Geometry: final body of the model. Coordinates: model frame, mm. Round coordinates to 2 decimals unless told otherwise and drop trailing zeros. Write each loop counter-clockwise with the first axis right and the second up, starting at its lowest first coordinate (ties: lowest second). Pieces come first, ordered by that corner, then holes. Notation, with made-up numbers: M 77.25,64 L 92.25,64 A33 cw 92.25,98 Z; hole C 27.5,77 d7. An arc over 180 degrees is marked long. Use one line per item in the form item = value. Start each with the question number.
Item 1: Section query A-A (z = 8.5). Return loops of the section in (x, y).
Item 2: Section query C-C (y = -6.5). Return loops of the section in (x, z), and give its area (3 significant figures).
Item 3: Pin query (flat end, axial travel): pin 1 Ø1 at (y, z) = (-99.5, 6) entering from -X; pin 2 Ø5 at (y, z) = (-77, 16) entering from +X; pin 3 Ø8 at (y, z) = (-72.5, 12) entering from -X. Return the tip coordinate at first contact, or that it passes through.
Item 4: Section query B-B (x = -91.5). Return loops of the section in (y, z).
Item 5: Ray query, probe 1 along Y at (x, z) = (108.5, 17); probe 2 along Y at (x, z) = (-93, 7.5); probe 3 along X at (y, z) = (-69, 2.25). Return the intervals inside material, ascending.
from build123d import *

# Parameters (mm, degrees)
BOSS_EXTRUDE1_DEPTH = 19.05
FILLET1_R           = 50.8


with BuildPart() as part:
    # Sketch1 → Boss-Extrude1 (new body)
    with BuildSketch(Plane.XY):
        with BuildLine():
            Line((-127, 0), (127, 0))
            Line((127, 0), (76.2, -101.6))
            ThreePointArc((76.2, -101.6), (0, -122.017728463), (-76.2, -101.6))
            Line((-76.2, -101.6), (-127, 0))
        make_face()
    extrude(amount=BOSS_EXTRUDE1_DEPTH)

    # Fillet1
    fillet1_edges = [part.edges().sort_by_distance(p)[0] for p in [
        (76.2, -101.6, 9.525),
        (-76.2, -101.6, 9.525),
    ]]
    fillet(fillet1_edges, radius=FILLET1_R)


solid = part.part
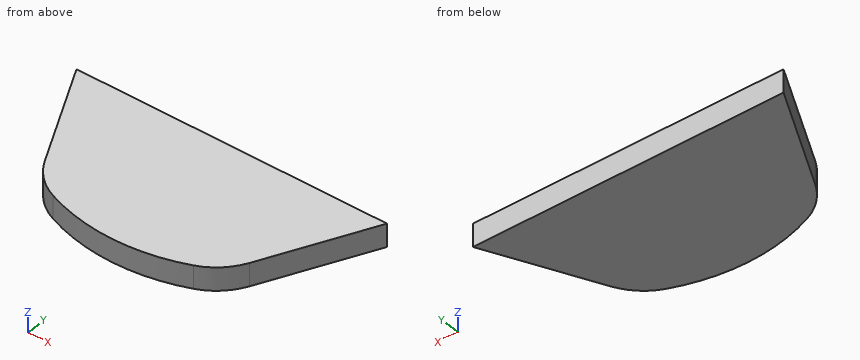
Working result:
q1.outline = M -127,0 L -83.79,-86.42 A50.8 ccw -57.53,-110.74 A152.4 ccw 57.53,-110.74 A50.8 ccw 83.79,-86.42 L 127,0 Z
q2.outline = M -123.75,0 L 123.75,0 L 123.75,19.05 L -123.75,19.05 Z
q2.area = 4,710 mm²
q3.pin_1 = -74.89
q3.pin_2 = 89.75
q3.pin_3 = -92.75
q4.outline = M -71,0 L 0,0 L 0,19.05 L -71,19.05 Z
q5.probe_1 = -37 to 0
q5.probe_2 = -68 to 0
q5.probe_3 = -92.5 to 92.5
